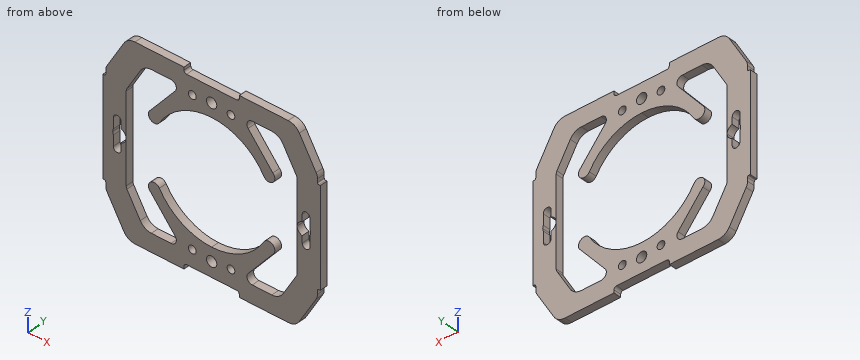
from build123d import *

# Parameters (mm, degrees)
F0_R     = 1.5
F0_R_2   = 2
F1_DEPTH = 3


with BuildPart() as f1:
    # F0 (on Front) → F1 (new body)
    with BuildSketch(Plane.XZ):
        with BuildLine():
            Line((41.110818, 19.5), (41.110818, 20.922697))
            ThreePointArc((41.110818, 20.922697), (40.973189, 21.962933), (40.569773, 22.931585))
            Line((40.569773, 22.931585), (34.076942, 34.11111))
            ThreePointArc((34.076942, 34.11111), (32.247687, 35.933333), (29.753248, 36.6))
            Line((29.753248, 36.6), (10.738378, 36.6))
            Line((10.738378, 36.6), (10.738378, 35.500753))
            ThreePointArc((10.738378, 35.500753), (10.445485, 34.793646), (9.738378, 34.500753))
            Line((9.738378, 34.500753), (0, 34.500753))
            Line((0, 34.500753), (-9.738378, 34.500753))
            ThreePointArc((-9.738378, 34.500753), (-10.445485, 34.793646), (-10.738378, 35.500753))
            Line((-10.738378, 35.500753), (-10.738378, 36.6))
            Line((-10.738378, 36.6), (-29.753248, 36.6))
            ThreePointArc((-29.753248, 36.6), (-32.247687, 35.933333), (-34.076942, 34.11111))
            Line((-34.076942, 34.11111), (-40.569773, 22.931585))
            ThreePointArc((-40.569773, 22.931585), (-40.973189, 21.962933), (-41.110818, 20.922697))
            Line((-41.110818, 20.922697), (-41.110818, 19.5))
            ThreePointArc((-41.110818, 19.5), (-41.257265, 19.146447), (-41.610818, 19))
            Line((-41.610818, 19), (-42.170605, 19))
            Line((-42.170605, 19), (-42.170605, 0))
            Line((-42.170605, 0), (-42.170605, -19))
            Line((-42.170605, -19), (-41.610818, -19))
            ThreePointArc((-41.610818, -19), (-41.257265, -19.146447), (-41.110818, -19.5))
            Line((-41.110818, -19.5), (-41.110818, -20.922697))
            ThreePointArc((-41.110818, -20.922697), (-40.973189, -21.962933), (-40.569773, -22.931585))
            Line((-40.569773, -22.931585), (-34.076942, -34.11111))
            ThreePointArc((-34.076942, -34.11111), (-32.247687, -35.933333), (-29.753248, -36.6))
            Line((-29.753248, -36.6), (-10.738378, -36.6))
            Line((-10.738378, -36.6), (-10.738378, -35.500753))
            ThreePointArc((-10.738378, -35.500753), (-10.445485, -34.793646), (-9.738378, -34.500753))
            Line((-9.738378, -34.500753), (0, -34.500753))
            Line((0, -34.500753), (9.738378, -34.500753))
            ThreePointArc((9.738378, -34.500753), (10.445485, -34.793646), (10.738378, -35.500753))
            Line((10.738378, -35.500753), (10.738378, -36.6))
            Line((10.738378, -36.6), (29.753248, -36.6))
            ThreePointArc((29.753248, -36.6), (32.247687, -35.933333), (34.076942, -34.11111))
            Line((34.076942, -34.11111), (40.569773, -22.931585))
            ThreePointArc((40.569773, -22.931585), (40.973189, -21.962933), (41.110818, -20.922697))
            Line((41.110818, -20.922697), (41.110818, -19.5))
            ThreePointArc((41.110818, -19.5), (41.257265, -19.146447), (41.610818, -19))
            Line((41.610818, -19), (42.170605, -19))
            Line((42.170605, -19), (42.170605, 0))
            Line((42.170605, 0), (42.170605, 19))
            Line((42.170605, 19), (41.610818, 19))
            ThreePointArc((41.610818, 19), (41.257265, 19.146447), (41.110818, 19.5))
        make_face()
        with Locations((-7.5, -28)):
            Circle(F0_R, mode=Mode.SUBTRACT)
        with Locations((0, -28.75)):
            Circle(F0_R_2, mode=Mode.SUBTRACT)
        with Locations((7.5, -28)):
            Circle(F0_R, mode=Mode.SUBTRACT)
        with BuildLine():
            ThreePointArc((-35.170605, 2.52267), (-33.751046, 1.600558), (-33.2, 0))
            ThreePointArc((-33.2, 0), (-33.751046, -1.600558), (-35.170605, -2.52267))
            Line((-35.170605, -2.52267), (-35.170605, -5.25))
            ThreePointArc((-35.170605, -5.25), (-36.670605, -6.75), (-38.170605, -5.25))
            Line((-38.170605, -5.25), (-38.170605, -1.067816))
            ThreePointArc((-38.170605, -1.067816), (-38.342004, -0.546089), (-38.4, 0))
            ThreePointArc((-38.4, 0), (-38.342004, 0.546089), (-38.170605, 1.067816))
            Line((-38.170605, 1.067816), (-38.170605, 5.25))
            ThreePointArc((-38.170605, 5.25), (-36.670605, 6.75), (-35.170605, 5.25))
            Line((-35.170605, 5.25), (-35.170605, 2.52267))
        make_face(mode=Mode.SUBTRACT)
        with Locations((-7.5, 28)):
            Circle(F0_R, mode=Mode.SUBTRACT)
        with BuildLine():
            ThreePointArc((23.368655, 29.672794), (25.863094, 29.006127), (27.692349, 27.183904))
            Line((27.692349, 27.183904), (32.890436, 18.233704))
            ThreePointArc((32.890436, 18.233704), (33.099337, 17.732107), (33.170605, 17.193441))
            Line((33.170605, 17.193441), (33.170605, 0))
            Line((33.170605, 0), (33.170605, -17.193441))
            ThreePointArc((33.170605, -17.193441), (33.099337, -17.732107), (32.890436, -18.233704))
            Line((32.890436, -18.233704), (27.692349, -27.183904))
            ThreePointArc((27.692349, -27.183904), (25.863094, -29.006127), (23.368655, -29.672794))
            Line((23.368655, -29.672794), (15.767856, -29.672794))
            ThreePointArc((15.767856, -29.672794), (13.892719, -28.480943), (14.175847, -26.2772))
            Line((14.175847, -26.2772), (23.769717, -14.746473))
            ThreePointArc((23.769717, -14.746473), (23.705468, -11.265364), (20.277872, -11.876781))
            ThreePointArc((20.277872, -11.876781), (11.686438, -20.388163), (0, -23.5))
            ThreePointArc((0, -23.5), (-11.686438, -20.388163), (-20.277872, -11.876781))
            ThreePointArc((-20.277872, -11.876781), (-23.705468, -11.265364), (-23.769717, -14.746473))
            Line((-23.769717, -14.746473), (-14.175847, -26.2772))
            ThreePointArc((-14.175847, -26.2772), (-13.892719, -28.480943), (-15.767856, -29.672794))
            Line((-15.767856, -29.672794), (-23.368655, -29.672794))
            ThreePointArc((-23.368655, -29.672794), (-25.863094, -29.006127), (-27.692349, -27.183904))
            Line((-27.692349, -27.183904), (-32.890436, -18.233704))
            ThreePointArc((-32.890436, -18.233704), (-33.099337, -17.732107), (-33.170605, -17.193441))
            Line((-33.170605, -17.193441), (-33.170605, 0))
            Line((-33.170605, 0), (-33.170605, 17.193441))
            ThreePointArc((-33.170605, 17.193441), (-33.099337, 17.732107), (-32.890436, 18.233704))
            Line((-32.890436, 18.233704), (-27.692349, 27.183904))
            ThreePointArc((-27.692349, 27.183904), (-25.863094, 29.006127), (-23.368655, 29.672794))
            Line((-23.368655, 29.672794), (-15.767856, 29.672794))
            ThreePointArc((-15.767856, 29.672794), (-13.892719, 28.480943), (-14.175847, 26.2772))
            Line((-14.175847, 26.2772), (-23.769717, 14.746473))
            ThreePointArc((-23.769717, 14.746473), (-23.705468, 11.265364), (-20.277872, 11.876781))
            ThreePointArc((-20.277872, 11.876781), (-11.686438, 20.388163), (0, 23.5))
            ThreePointArc((0, 23.5), (11.686438, 20.388163), (20.277872, 11.876781))
            ThreePointArc((20.277872, 11.876781), (23.705468, 11.265364), (23.769717, 14.746473))
            Line((23.769717, 14.746473), (14.175847, 26.2772))
            ThreePointArc((14.175847, 26.2772), (13.892719, 28.480943), (15.767856, 29.672794))
            Line((15.767856, 29.672794), (23.368655, 29.672794))
        make_face(mode=Mode.SUBTRACT)
        with BuildLine():
            ThreePointArc((35.170605, -2.52267), (33.751046, -1.600558), (33.2, 0))
            ThreePointArc((33.2, 0), (33.751046, 1.600558), (35.170605, 2.52267))
            Line((35.170605, 2.52267), (35.170605, 5.25))
            ThreePointArc((35.170605, 5.25), (36.670605, 6.75), (38.170605, 5.25))
            Line((38.170605, 5.25), (38.170605, 1.067816))
            ThreePointArc((38.170605, 1.067816), (38.342004, 0.546089), (38.4, 0))
            ThreePointArc((38.4, 0), (38.342004, -0.546089), (38.170605, -1.067816))
            Line((38.170605, -1.067816), (38.170605, -5.25))
            ThreePointArc((38.170605, -5.25), (36.670605, -6.75), (35.170605, -5.25))
            Line((35.170605, -5.25), (35.170605, -2.52267))
        make_face(mode=Mode.SUBTRACT)
        with Locations((0, 28.75)):
            Circle(F0_R_2, mode=Mode.SUBTRACT)
        with Locations((7.5, 28)):
            Circle(F0_R, mode=Mode.SUBTRACT)
    extrude(amount=F1_DEPTH)


solid = f1.part
For this review, take the finished solid that the model builds, in its own axes (mm). Round coordinates to 2 decimals unless told otherwise and drop trailing zeros. Order: outer loops, then holes, each group sorted by start corner. A loop starts at its lowest first (then second) coordinate and runs counter-clockwise, first axis right, second up. Notation, with made-up numbers: (-16.5, 47) -> (-6.5, 47) arc R21 cw to (-6.5, 63) -> close; hole circle Ø3 at (74, -39.5). An arc over 180 degrees is marked (long way). Put each result on its own line as item: value.
Q1. Add section C-C on y = -0.75. State how many separate pieces and enclosed holes the cut face has, plus the area to 3 significant figures.
Check result:
separate pieces: 1
enclosed holes: 9
area: 2,530 mm2
Q2. Insertion check: pin 1 Ø1.1 at (y, z) = (-2, -20.5) entering from -X; pin 2 Ø2.5 at (x, z) = (7.5, -28) entering from +Y. Each pin has a flat end and moves straight along its axis. Give the tip position at first contact, or say it passes through.
Check result:
pin 1: x = -41.11
pin 2: through
Q3. Add section B-B on x = 7.5. Write out the cut boundary in (y, z), plus the area to 3 significant figures.
Check result:
outline: (-3, -34.5) -> (0, -34.5) -> (0, -29.5) -> (-3, -29.5) -> close; (-3, -26.5) -> (0, -26.5) -> (0, -22.27) -> (-3, -22.27) -> close; (-3, 22.27) -> (0, 22.27) -> (0, 26.5) -> (-3, 26.5) -> close; (-3, 29.5) -> (0, 29.5) -> (0, 34.5) -> (-3, 34.5) -> close
area: 55.4 mm2
Q4. Add section A-A on x = 31. Write out the cut boundary in (y, z), plus the area to 3 significant figures.
Check result:
outline: (-3, -36.44) -> (0, -36.44) -> (0, -21.49) -> (-3, -21.49) -> close; (-3, 21.49) -> (0, 21.49) -> (0, 36.44) -> (-3, 36.44) -> close
area: 89.7 mm2
Q5. For probe 1 along Z at (x, y) = (-7.5, -1.15); probe 2 along X at (y, z) = (-0.8, 12); probe 3 along Z at (x, y) = (-14, -1.2), list the stretches that pass through material, from the lowest coordinate up. Write a range as [from, to].
Check result:
probe 1: [-34.5, -29.5], [-26.5, -22.27], [22.27, 26.5], [29.5, 34.5]
probe 2: [-42.17, -33.17], [-24.29, -20.21], [20.21, 24.29], [33.17, 42.17]
probe 3: [-36.6, -28.68], [-26.52, -18.87], [18.87, 26.52], [28.68, 36.6]
